```python
from build123d import *

# Parameters (mm, degrees)
BOSS_EXTRUDE1_DEPTH         = 2
SKETCH4_R                   = 7
BOSS_EXTRUDE2_DEPTH         = 2
M12X1_25_TAPPED_HOLE2_D     = 10.8
M12X1_25_TAPPED_HOLE2_DEPTH = 8.75
M12X1_25_TAPPED_HOLE2_TIP   = 3.244647343


with BuildPart() as part:
    # Sketch1 → Boss-Extrude1 (new body)
    with BuildSketch(Plane.XY):
        Polygon((-7.272664144, 4.028443403), (-7.125066396, -4.284090201), (0.147597748, -8.312533603), (7.272664144, -4.028443403), (7.125066396, 4.284090201), (-0.147597748, 8.312533603), align=None)
    extrude(amount=BOSS_EXTRUDE1_DEPTH)

    # Sketch4 → Boss-Extrude2 (add)
    with BuildSketch(Plane.XY.offset(2)):
        Circle(SKETCH4_R)
    extrude(amount=BOSS_EXTRUDE2_DEPTH)

    # M12x1.25 Tapped Hole2
    with Locations(Plane.XY.offset(4)):
        with Locations((0, 0)):
            Hole(M12X1_25_TAPPED_HOLE2_D / 2, depth=M12X1_25_TAPPED_HOLE2_DEPTH)
            with Locations((0, 0, -(M12X1_25_TAPPED_HOLE2_DEPTH + M12X1_25_TAPPED_HOLE2_TIP / 2))):  # 118° drill point
                Cone(0, M12X1_25_TAPPED_HOLE2_D / 2, M12X1_25_TAPPED_HOLE2_TIP, mode=Mode.SUBTRACT)


solid = part.part
```
The listing builds one solid part. Answer for the finished solid, in the listing's coordinates (mm). A direction names the side the tool comes from. Give positions to 0.01 mm unless a question says otherwise; leave off trailing zeros. Order: outer loops, then holes, each group sorted by start corner. A loop starts at its lowest first (then second) coordinate and runs counter-clockwise, first axis right, second up. Notation, with made-up numbers: (-27.5, -31) -> (22.5, -31) arc R23 cw to (22.5, -14) -> close; hole circle Ø7 at (-35.5, 82.25). An arc over 180 degrees is marked (long way). Write each question's results on one line, items separated by ' | '.
Q1. Each of these flat-tipped pins is pushed along its axis until it touches: P1, Ø2, axis at x = -2.5, z = 2.5, coming from the +Y side; P2, Ø1, axis at x = -5.5, z = 3, coming from the +Y side. Where does it stop, or does it pass through?
Checked values:
P1: stops at y = 7.42 | P2: stops at y = 4.9
Q2. Straight lines are drawn through the part: probe 1 along Y at (x, z) = (0, 2.75); probe 2 along Y at (x, z) = (0, 0.45); probe 3 along X at (y, z) = (-2.5, 2.45). For each, find the intervals that lie inside material, in ascending order. Write a range as from..to.
Checked values:
probe 1: y = -7..-5.4, 5.4..7 | probe 2: y = -8.23..-5.4, 5.4..8.23 | probe 3: x = -6.54..-4.79, 4.79..6.54
Q3. Determine the mould class of faces 1 (the face through (-1.7, -5.4, 0)), 2 (the face through (3.66, -6.2, 0.99)), 3 (the face through (1.17, -5.27, 1.97)), 4 (the face through (-3.54, -6.27, 0.99)) for opening direction X: pulls with the +X half, pulls with the -X half, needs draft (parallel to the pull), parting line crosses it, or undercut.
Checked values:
face 1: needs draft | face 2: pulls with the +X half | face 3: undercut | face 4: pulls with the -X half
Q4. The part is cut by section B-B, the plane y = 2. Give the vertices of the cut face in (x, z), and give its area (3 significant figures).
Checked values:
outline: (-7.24, 0) -> (-5.02, 0) -> (-5.02, 4) -> (-6.71, 4) -> (-6.71, 2) -> (-7.24, 2) -> close; (5.02, 0) -> (7.17, 0) -> (7.17, 2) -> (6.71, 2) -> (6.71, 4) -> (5.02, 4) -> close | area: 15.5 mm^2
Q5. Which of the six approach directions +Z, -Z, +X, -X, +Y, -Y give full straight-line access (tool end or side, diameter ignored) to faces 5 (the face through (3.54, 6.27, 0.99)), 6 (the face through (6.466, -2.681, 2.986))?
Checked values:
face 5: +Z, -Z, +X, +Y | face 6: +Z
Q6. The part is cut by section C-C, the plane x = -4.75. Give the vertices of the cut face in (y, z).
Checked values:
outline: (-5.6, 0) -> (-2.57, 0) -> (-2.57, 4) -> (-5.14, 4) -> (-5.14, 2) -> (-5.6, 2) -> close; (2.57, 0) -> (5.55, 0) -> (5.55, 2) -> (5.14, 2) -> (5.14, 4) -> (2.57, 4) -> close
Q7. The part is cut by section D-D, the plane y = 6.5. Give the vertices of the cut face in (x, z), and give its area (3 significant figures).
Checked values:
outline: (-3.16, 0) -> (3.12, 0) -> (3.12, 2) -> (2.6, 2) -> (2.6, 4) -> (-2.6, 4) -> (-2.6, 2) -> (-3.16, 2) -> close | area: 23.0 mm^2
Q8. The part is cut by section A-A, the plane z = 1.55. Give the vertices of the cut face in (x, y), and give its area (3 significant figures).
Checked values:
outline: (-7.27, 4.03) -> (-7.13, -4.28) -> (0.15, -8.31) -> (7.27, -4.03) -> (7.13, 4.28) -> (-0.15, 8.31) -> close; hole circle Ø10.8 at (0, 0) | area: 88.0 mm^2
